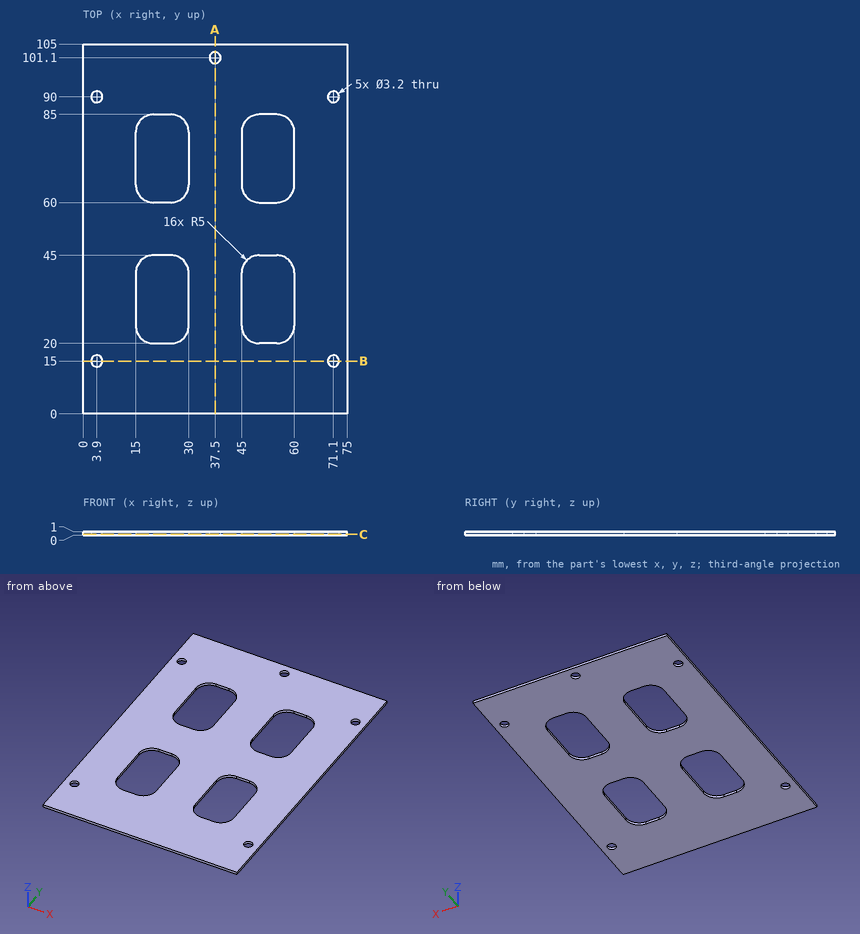
Study the drawing (mm; zero at the part's minimum x, y, z) and answer. Give positions to 0.01 mm unless a question says otherwise; leave off trailing zeros. Loops run counter-clockwise (first coordinate to the right, second up) from the corner with the lowest first, then second, coordinate; pieces in that order, holes last. Notation, with made-up numbers: M 19.5,15 L 62.5,15 A25 ccw 62.5,46 Z; hole C 52,-19.5 d8. An arc over 180 degrees is marked long. Answer as CSV lines item,"result".
Item 1: Given pin 1 Ø2.5 at (x, y) = (37.5, 101.1) entering from -Z, flat-ended and moving along its own axis, determine where the tip first touches the part or whether it passes through.
Values follow:
pin 1,"passes through"
Item 2: The part is cut by section A-A (x = 37.5). Give the vertices of the cut face in (y, z).
Values follow:
outline,"M 0,0 L 99.5,0 L 99.5,1 L 0,1 Z; M 102.7,0 L 105,0 L 105,1 L 102.7,1 Z"
Item 3: The part is cut by section C-C (z = 0.3). Give the number of separate pieces and of enclosed holes in the cut face, and give its area (3 significant figures).
Values follow:
separate pieces,"1"
enclosed holes,"9"
area,"6,420 mm^2"
Item 4: Straight lines are drawn through the part: line 1 along X through (y, z) = (29, 0.3); line 2 along Y through (x, z) = (71.1, 0.7); line 3 along Y through (x, z) = (37.5, 0.75). For each, find the intervals that lie inside material, in ascending order. Write a range as [from, to].
Values follow:
line 1,"x = [0, 15], [30, 45], [60, 75]"
line 2,"y = [0, 13.4], [16.6, 88.4], [91.6, 105]"
line 3,"y = [0, 99.5], [102.7, 105]"
Item 5: The part is cut by section B-B (y = 15). Give the vertices of the cut face in (x, z), and give its area (3 significant figures).
Values follow:
outline,"M 0,0 L 2.3,0 L 2.3,1 L 0,1 Z; M 5.5,0 L 69.5,0 L 69.5,1 L 5.5,1 Z; M 72.7,0 L 75,0 L 75,1 L 72.7,1 Z"
area,"68.6 mm^2"
